from build123d import *

# Parameters (mm, degrees)
BOSS_EXTRUDE1_DEPTH      = 16.5
BOSS_EXTRUDE1_DEPTH_BACK = 16.5
SKETCH1_W                = 30
SKETCH1_H                = 175
SKETCH2_R                = 9
CUT_EXTRUDE1_DEPTH       = 3
FILLET1_R                = 15
SKETCH3_R                = 4
CUT_EXTRUDE2_DEPTH       = 4
DRAFT1_ANGLE             = -2


with BuildPart() as part:
    # Sketch1 → Boss-Extrude1 (new, two sides: drawn at the far end of the back side and taken through both)
    with BuildSketch(Plane(origin=(0, 0, 0), x_dir=(0, 0, -1), z_dir=(1, 0, 0)).offset(-BOSS_EXTRUDE1_DEPTH_BACK)):
        Rectangle(SKETCH1_W, SKETCH1_H)
    extrude(amount=BOSS_EXTRUDE1_DEPTH + BOSS_EXTRUDE1_DEPTH_BACK)

    # Sketch2 → Cut-Extrude1 (cut)
    with BuildSketch(Plane(origin=(16.5, 0, 0), x_dir=(0, 0, -1), z_dir=(1, 0, 0))):
        with Locations((0, -60)):
            Circle(SKETCH2_R)
        with Locations((0, 60)):
            Circle(SKETCH2_R)
    extrude(amount=-CUT_EXTRUDE1_DEPTH, mode=Mode.SUBTRACT)

    # Fillet1
    fillet1_edges = [part.edges().sort_by_distance(p)[0] for p in [
        (0, 87.5, -15),
        (0, 87.5, 15),
        (0, -87.5, -15),
        (0, -87.5, 15),
    ]]
    fillet(fillet1_edges, radius=FILLET1_R - 0.0001)  # a hair under: the kernel refuses the full size

    # Sketch3 → Cut-Extrude2 (cut)
    with BuildSketch(Plane(origin=(0, 0, -15), x_dir=(-1, 0, 0), z_dir=(0, 0, -1))):
        with Locations((-0.6, 0)):
            Circle(SKETCH3_R)
    extrude(amount=-CUT_EXTRUDE2_DEPTH, mode=Mode.SUBTRACT)

    # Draft1
    draft1_faces = [part.faces().sort_by_distance(p)[0] for p in [
        (0, -83.106631007, -10.606631007),
        (15.012920379, 0, -15),
        (0, 83.106631007, -10.606631007),
        (0, 83.106631007, 10.606631007),
        (0, 0, 15),
        (0, -83.106631007, 10.606631007),
    ]]
    draft(draft1_faces, Plane(origin=(-16.5, 0, 0), x_dir=(0, 0, -1), z_dir=(-1, 0, 0)), DRAFT1_ANGLE)


solid = part.part
Could you check a few things on this model? Use its own coordinates, in mm. A direction names the side the tool comes from. Coordinates: 2 decimals unless noted, no trailing zeros. Loops run counter-clockwise (first coordinate to the right, second up) from the corner with the lowest first, then second, coordinate; pieces in that order, holes last. Notation, with made-up numbers: (-11.5, -20) -> (11.5, -20) arc R15 cw to (11.5, -12) -> close; hole circle Ø2 at (-30, 56). An arc over 180 degrees is marked (long way). Answer in a Markdown table with one row per item.
(1) Imagine slicing it at D-D (y = 31.5). List the corners of the cut face in (x, z) for me.
Results found:
| item | result |
|---|---|
| outline | (-16.5, -15) -> (16.5, -13.85) -> (16.5, 13.85) -> (-16.5, 15) -> close |
(2) Imagine slicing it at A-A (y = -60). List the corners of the cut face in (x, z) for me.
Results found:
| item | result |
|---|---|
| outline | (-16.5, -15) -> (16.5, -13.85) -> (16.5, -9) -> (13.5, -9) -> (13.5, 9) -> (16.5, 9) -> (16.5, 13.85) -> (-16.5, 15) -> close |
(3) For faces 1 (the face through (0.231, 82.805, -10.081)), 2 (the face through (13.5, -60, 0)), 3 (the face through (1, 0, -11)), which set-ups out of +Z, -Z, +X, -X, +Y, -Y let a thin tool reach every point of the face, with its end or its side?
Results found:
| item | result |
|---|---|
| face 1 | -Z, +X, +Y |
| face 2 | +X |
| face 3 | -Z |
(4) If I drill on probe 1 along Y at (x, z) = (14, 0); probe 2 along Z at (x, y) = (14.5, -63.5); probe 3 along X at (y, z) = (-60.5, 8.5), over which ranges is the centre line in solid material (lowest first)?
Results found:
| item | result |
|---|---|
| probe 1 | y = -86.43 to -69, -51 to 51, 69 to 86.43 |
| probe 2 | z = -13.92 to -8.29, 8.29 to 13.92 |
| probe 3 | x = -16.5 to 13.5 |
(5) Thinking about a two-plate mould opening in Y: for faces 4 (the face through (-16.5, 1, 0)), 5 (the face through (0.231, -82.805, -10.081)), 6 (the face through (13.5, 60, 0)), which applies, released by +Y, released by -Y, zero draft, split by the parting line, or undercut?
Results found:
| item | result |
|---|---|
| face 4 | zero draft |
| face 5 | released by -Y |
| face 6 | undercut |
(6) Will these pins go through, and if not, where does the flat tip stop? pin 1 Ø5 at (x, y) = (-11.5, 15) entering from +Z; pin 2 Ø5.5 at (y, z) = (-60, -3.5) entering from +X; pin 3 Ø6 at (x, z) = (7.5, 3.5) entering from +Y.
Results found:
| item | result |
|---|---|
| pin 1 | stops at z = 14.91 |
| pin 2 | stops at x = 13.5 |
| pin 3 | stops at y = 86.69 |
